```python
from build123d import *

# Parameters (mm, degrees)
F0_R      = 1.5
F1_DEPTH  = 3
F2_W      = 18.5
F2_H      = 6.625
F3_DEPTH  = 25
F4_W      = 18.5
F4_H      = 9
F5_DEPTH  = 1
F6_DEPTH  = 2
F8_D      = 1.6
F9_SIZE   = 0.99999
F10_W     = 6
F10_H     = 6
F11_DEPTH = 8
F12_R     = 2.99999
F13_W     = 6
F13_H     = 6
F14_DEPTH = 8
F15_R     = 2.99999
F17_D     = 2.5
F18_R     = 0.5
F19_DEPTH = 9.625


# Not quite as in the source:
# - a fillet or chamfer is up to 0.001 mm smaller than in the source, because OpenCascade refuses the exact size


with BuildPart() as f1:
    # F0 (on Right) → F1 (new body)
    with BuildSketch(Plane.YZ):
        with BuildLine():
            Line((-64, -8), (10, -8))
            Line((10, -8), (10, 5))
            Line((10, 5), (20, 5))
            add(Edge.make_bspline(
                [(-65.5, 29), (-53.1884357333, 31.5765216947), (-28.2810822655, 35.0271902112), (17.668255518, 10.972023372), (20, 5)],
                knots=[0, 0, 0, 0, 0.471377868, 1, 1, 1, 1], degree=3))
            Line((-65.5, 29), (-62, 25))
            Line((-62, 25), (-71.3544447211, 3.1483555777))
            ThreePointArc((-71.3544447211, 3.1483555777), (-70.677830659, -4.4052897395), (-64, -8))
        make_face()
        with Locations((-64, 0)):
            Circle(F0_R, mode=Mode.SUBTRACT)
        Circle(F0_R, mode=Mode.SUBTRACT)
        with Locations((-49, 19)):
            Circle(F0_R, mode=Mode.SUBTRACT)
    extrude(amount=F1_DEPTH)

    # F2 (on face) → F3 (cut)
    with BuildSketch(Plane.YZ.offset(3)):
        with Locations((-32, 3.3125)):
            Rectangle(F2_W, F2_H)
        with Locations((-32, -3.3125)):
            Rectangle(F2_W, F2_H)
    extrude(amount=-F3_DEPTH, mode=Mode.SUBTRACT)

    # F4 (on face) → F5 (join)
    with BuildSketch(Plane(origin=(0, 0, 0), x_dir=(0, -1, 0), z_dir=(-1, 0, 0))):
        with Locations((32, 2.125)):
            Rectangle(F4_W, F4_H)
        Polygon((42.25, -2.375), (42.25, 7.625), (21.75, 7.625), (21.75, -2.375), (22.75, -2.375), (22.75, 6.625), (41.25, 6.625), (41.25, -2.375), align=None)
    extrude(amount=F5_DEPTH)

    # F6 (add): a face of the model
    f6_faces = [f1.faces().sort_by_distance(p)[0] for p in [
        (0, -32, 2.125),
    ]]
    extrude(f6_faces, amount=F6_DEPTH)

    # F8 (through all)
    with Locations(Plane.YZ.offset(2)):
        with Locations((-38.35, 3.775), (-25.65, 3.775)):
            Hole(F8_D / 2)

    # F9 (size 1 in the source; OpenCascade refuses exactly that, so slightly less here)
    f9_edges = [f1.edges().sort_by_distance(p)[0] for p in [
        (-1, -21.75, 2.625),
        (-1, -42.25, 2.625),
    ]]
    chamfer(f9_edges, length=F9_SIZE)

    # F10 (on face) → F11 (join)
    with BuildSketch(Plane(origin=(0, 0, 0), x_dir=(0, -1, 0), z_dir=(-1, 0, 0))):
        with Locations((49, 4.625)):
            Rectangle(F10_W, F10_H)
    extrude(amount=F11_DEPTH)

    # F12 (radius 3 in the source; OpenCascade refuses exactly that, so slightly less here)
    f12_edges = [f1.edges().sort_by_distance(p)[0] for p in [
        (-8, -52, 4.625),
        (-8, -46, 4.625),
    ]]
    fillet(f12_edges, radius=F12_R)

    # F13 (on face) → F14 (join)
    with BuildSketch(Plane(origin=(0, 0, 0), x_dir=(0, -1, 0), z_dir=(-1, 0, 0))):
        with Locations((15, 4.625)):
            Rectangle(F13_W, F13_H)
    extrude(amount=F14_DEPTH)

    # F15 (radius 3 in the source; OpenCascade refuses exactly that, so slightly less here)
    f15_edges = [f1.edges().sort_by_distance(p)[0] for p in [
        (-8, -12, 4.625),
        (-8, -18, 4.625),
    ]]
    fillet(f15_edges, radius=F15_R)

    # F17 (through all)
    with Locations(Plane.XY.offset(7.625)):
        with Locations((-5, -49), (-5, -15)):
            Hole(F17_D / 2)

    # F18
    f18_edges = [f1.edges().sort_by_distance(p)[0] for p in [
        (1.5, -65.5, 29),
        (1.5, 20, 5),
    ]]
    fillet(f18_edges, radius=F18_R)

    # F19 (add): faces of the model
    f19_faces = [f1.faces().sort_by_distance(p)[0] for p in [
        (-3.5469743881, -15, 1.625),
        (-3.5469743881, -49, 1.625),
    ]]
    extrude(f19_faces, amount=F19_DEPTH)


solid = f1.part
```
For this review, take the finished solid that the model builds, in its own axes (mm). A direction names the side the tool comes from. Give positions to 0.01 mm unless a question says otherwise; leave off trailing zeros.
Item 1: The part is to be moulded in two halves that separate along Y. For faces 1 (the face through (0.48, -37.55, 3.81)), 2 (the face through (-2, -12, 0)), 3 (the face through (1.48, -63.49, 26.7)), 4 (the face through (1, -26, -8)), say which applies: +Y half, -Y half, draft (parallel to the pull), parting line (faces both ways), or undercut.
Item 2: Take a section at A-A (x = 1). Give the number of separate pieces and of enclosed holes in the cut face, and give its area (3 significant figures).
Item 3: Wall thickness on probe 1 along Y at (x, z) = (-5, -2); probe 2 along Z at (x, y) = (1.5, -64); probe 3 along Z at (x, y) = (-0.1, -25.65) (3 decimals): over which ranges is each line inside the solid? List them lowest first.
Item 4: Insertion check: P1, Ø5.5, axis at x = -3, z = -2.5, coming from the -Y side; P2, Ø4, axis at y = 0, z = 0, coming from the +X side; P3, Ø3, axis at y = -22.5, z = 0.5, coming from the -X side; P4, Ø4.5, axis at y = -30.5, z = 3, coming from the +X side. Each pin has a flat end and moves straight along its axis. Give the tip position at first contact, or say it passes through.
Item 5: Machinability: for faces 5 (the face through (-1, -32, 3)), 6 (the face through (-2, -52, 0)), 7 (the face through (1, 15, 5)), 8 (the face through (-3, -15, 7.625)), 9 (the face through (2.2, -22.75, -1.6)), which of the approach directions +Z, -Z, +X, -X, +Y, -Y give a long, thin tool a straight path to every point of the face, cutting with its end or side? Answer none if there is none.
Established:
1. face 1: undercut
1. face 2: +Y half
1. face 3: -Y half
1. face 4: draft
2. separate pieces: 1
2. enclosed holes: 6
2. area: 2,640 mm2
3. probe 1: y = -52 to -50.25, -47.75 to -46, -18 to -16.25, -13.75 to -12
3. probe 2: z = -8 to -1.5, 1.5 to 20.33, 27.29 to 29.31
3. probe 3: z = -2.375 to 2.975, 4.575 to 7.625
4. P1: stops at y = -52
4. P2: stops at x = 3
4. P3: stops at x = -1
4. P4: stops at x = 2
5. face 5: +Z, -Z, -X
5. face 6: +Z, -Z, -X, -Y
5. face 7: -Z, +X, -X, +Y
5. face 8: +Z, -X, +Y, -Y
5. face 9: +X
